Work out the finished part from the listing and answer in its coordinate system (mm). A direction names the side the tool comes from. Coordinates: 2 decimals unless noted, no trailing zeros. Order: outer loops, then holes, each group sorted by start corner. A loop starts at its lowest first (then second) coordinate and runs counter-clockwise, first axis right, second up. Notation, with made-up numbers: (-29, 29) - (-14, 29) arc R22 cw to (-14, 41) - close; hole circle Ø8 at (62.25, 33.25). An arc over 180 degrees is marked (long way). Answer as a JSON object with one key per item and string values. Group by question number.
1) Each of these flat-tipped pins is pushed along its axis until it touches: P1, Ø6, axis at x = 65.5, y = -100.5, coming from the -Z side; P2, Ø3, axis at y = -25, z = 13.5, coming from the -X side; P3, Ø1, axis at y = -171.5, z = 15, coming from the -X side; P4, Ø10, axis at y = -170, z = 19, coming from the -X side. Where does it stop, or does it pass through?
2) Section B-B (z = 16) is taken. Count the separate pieces of the cut face and the enclosed holes in it, plus the area to 3 significant figures.
3) A tool of negligible diameter and unlimited length cuts with its end or side. For faces 5 (the face through (9.835, -152.117, 11.268)), 6 (the face through (2.4, -100.2, 11.3)), from which of +Z, -Z, +X, -X, +Y, -Y can it reach the whole face along a straight path? Write none if from no direction.
4) The mould has two halves that part along Y. Classify faces 1 (the face through (9.81, -50.51, 11.27)), 2 (the face through (71.117, -51.079, 11.268)), 3 (the face through (38, 0, 11)), 4 (the face through (76.2, -100, 11)): released by +Y, released by -Y, zero draft, split by the parting line, or undercut.
5) Section A-A (y = -149) is taken. Give the vertices of the cut face in (x, z) (3 decimals).
6) Section C-C (x = 24.5) is taken. Give the vertices of the cut face in (y, z) (1 decimal), plus the area to 3 significant figures.
7) Section D-D (x = 40.5) is taken. Give the vertices of the cut face in (y, z) (3 decimals), plus the area to 3 significant figures.
8) Find the intervals of material crossed by line 1 along Y through (x, z) = (44.5, 4.25); line 2 along Y through (x, z) = (62, 18.25); line 3 along X through (y, z) = (-42.5, 18), in increasing order.
from build123d import *

# Parameters (mm, degrees)
F1_DEPTH = 203.2
F2_DEPTH = 203.2
F4_DEPTH = 25.4


with BuildPart() as f1:
    # F0 (on Front) → F1 (new body)
    with BuildSketch(Plane.XZ):
        Polygon((4.7240695831, 22.225), (0, 0), (76.2, 0), (76.2, 22.225), align=None)
    extrude(amount=F1_DEPTH)

    # F0 (on Front) → F2 (join)
    with BuildSketch(Plane.XZ):
        Polygon((4.7240695831, 22.225), (0, 0), (76.2, 0), (76.2, 22.225), align=None)
    extrude(amount=F2_DEPTH)

    # F3 (on face) → F4 (cut)
    with BuildSketch(Plane.XY.offset(22.225)):
        with BuildLine():
            ThreePointArc((22.500173924, -63.4888712894), (9.8102666247, -50.7932735364), (22.5036881615, -38.1011894183))
            ThreePointArc((22.5036881615, -38.1011894183), (9.8080901072, -50.7932732351), (22.500173924, -63.4888712894))
        make_face()
        with BuildLine():
            Line((58.4195802106, -38.1000022454), (22.5036881615, -38.1011894183))
            ThreePointArc((22.5036881615, -38.1011894183), (9.8102666247, -50.7932735364), (22.500173924, -63.4888712894))
            Line((22.500173924, -63.4888712894), (58.416064268, -63.5000016286))
            ThreePointArc((58.416064268, -63.5000016286), (58.4178222393, -63.5000020517), (58.4195802106, -63.5000022315))
            ThreePointArc((58.4195802106, -63.5000022315), (71.1199999996, -50.8000022384), (58.4195802106, -38.1000022454))
        make_face()
        with BuildLine():
            Line((58.4195802106, -89.2484490539), (22.501472381, -89.2484490539))
            ThreePointArc((22.501472381, -89.2484490539), (9.9718902315, -101.7780312034), (22.501472381, -114.3076133529))
            Line((22.501472381, -114.3076133529), (58.4195802106, -114.3076133529))
            ThreePointArc((58.4195802106, -114.3076133529), (70.9491623601, -101.7780312034), (58.4195802106, -89.2484490539))
        make_face()
        with BuildLine():
            Line((58.4111609952, -139.7000054607), (22.4953197832, -139.7250023393))
            ThreePointArc((22.4953197832, -139.7250023393), (9.8321170384, -152.3959699434), (22.4932164886, -165.0690392045))
            Line((22.4932164886, -165.0690392045), (58.4090530569, -165.0999973742))
            ThreePointArc((58.4090530569, -165.0999973742), (58.4143166333, -165.1000008204), (58.4195802107, -165.1000020852))
            ThreePointArc((58.4195802107, -165.1000020852), (71.1199998532, -152.4000022384), (58.4195802107, -139.7000023917))
            ThreePointArc((58.4195802107, -139.7000023917), (58.4153706027, -139.7000032285), (58.4111609952, -139.7000054607))
        make_face()
    extrude(amount=-F4_DEPTH, mode=Mode.SUBTRACT)


solid = f1.part
Report:
{
 "1": {"P1": "passes through", "P2": "stops at x = 2.55", "P3": "stops at x = 3.08", "P4": "stops at x = 2.98"},
 "2": {"separate pieces": "1", "enclosed holes": "3", "area": "10,600 mm²"},
 "3": {"face 5": "+Z, -Z", "face 6": "+Z, -X, +Y, -Y"},
 "4": {"face 1": "undercut", "face 2": "undercut", "face 3": "released by +Y", "face 4": "zero draft"},
 "5": {"outline": "(0, 0) - (10.296, 0) - (10.296, 22.225) - (4.724, 22.225) - close; (70.656, 0) - (76.2, 0) - (76.2, 22.225) - (70.656, 22.225) - close"},
 "6": {"outline": "(-203.2, 0) - (-165.1, 0) - (-165.1, 22.2) - (-203.2, 22.2) - close; (-139.7, 0) - (-114.3, 0) - (-114.3, 22.2) - (-139.7, 22.2) - close; (-89.2, 0) - (-63.5, 0) - (-63.5, 22.2) - (-89.2, 22.2) - close; (-38.1, 0) - (0, 0) - (0, 22.2) - (-38.1, 22.2) - close", "area": "2,830 mm²"},
 "7": {"outline": "(-203.2, 0) - (-165.085, 0) - (-165.085, 22.225) - (-203.2, 22.225) - close; (-139.712, 0) - (-114.308, 0) - (-114.308, 22.225) - (-139.712, 22.225) - close; (-89.248, 0) - (-63.494, 0) - (-63.494, 22.225) - (-89.248, 22.225) - close; (-38.101, 0) - (0, 0) - (0, 22.225) - (-38.101, 22.225) - close", "area": "2,830 mm²"},
 "8": {"line 1": "y = -203.2 to -165.09, -139.71 to -114.31, -89.25 to -63.5, -38.1 to 0", "line 2": "y = -203.2 to -164.58, -140.22 to -113.79, -89.77 to -62.98, -38.62 to 0", "line 3": "x = 3.83 to 12.89, 68.03 to 76.2"}
}
